Work out the finished part from the listing and answer in its coordinate system (mm). A direction names the side the tool comes from. Round coordinates to 2 decimals unless told otherwise and drop trailing zeros. Loops run counter-clockwise (first coordinate to the right, second up) from the corner with the lowest first, then second, coordinate; pieces in that order, holes last. Notation, with made-up numbers: (-27, 65) - (-6, 65) arc R17 ccw to (-6, 92) - close; hole circle Ø6 at (-24, 76). An arc over 180 degrees is marked (long way). Return JSON: item names as keys, results as strings.
from build123d import *

# Parameters (mm, degrees)
SKETCH1_R           = 7.85
SKETCH1_R_2         = 1.5625
SKETCH1_R_3         = 2
BOSS_EXTRUDE1_DEPTH = 4.7625
BOSS_EXTRUDE2_DEPTH = 4.7625
SKETCH4_R           = 2
SKETCH4_W           = 5.5
SKETCH4_H           = 17.5
CUT_EXTRUDE1_DEPTH  = 5.7625
CHAMFER1_SIZE       = 3
FILLET1_R           = 4.5
FILLET2_R           = 2


with BuildPart() as part:
    # Sketch1 → Boss-Extrude1 (new body)
    with BuildSketch(Plane(origin=(0, 0, 0), x_dir=(1, 0, 0), z_dir=(0, 1, 0))):
        with BuildLine():
            Line((-36.456035166, 71.322980167), (-35.908059548, 74.43070433))
            ThreePointArc((-35.908059548, 74.43070433), (-34.303826486, 77.194114594), (-34.866170482, 80.339550848))
            Line((-34.866170482, 80.339550848), (-33.339099631, 89))
            Line((-33.339099631, 89), (-28, 89))
            ThreePointArc((-28, 89), (-25, 87.9), (-22, 89))
            Line((-22, 89), (-16.5, 89))
            Line((-16.5, 89), (-7.269449675, 79.769449675))
            ThreePointArc((-7.269449675, 79.769449675), (0, 80.1), (7.269449675, 79.769449675))
            Line((7.269449675, 79.769449675), (16.5, 89))
            Line((16.5, 89), (22, 89))
            ThreePointArc((22, 89), (25, 87.9), (28, 89))
            Line((28, 89), (33.339099631, 89))
            Line((33.339099631, 89), (34.866170482, 80.339550848))
            ThreePointArc((34.866170482, 80.339550848), (34.303826486, 77.194114594), (35.908059548, 74.43070433))
            Line((35.908059548, 74.43070433), (36.456035166, 71.322980167))
            ThreePointArc((36.456035166, 71.322980167), (43.225467457, 67.435665364), (49.584363344, 62.907876389))
            Line((49.584363344, 62.907876389), (83.633453422, 92.871075657))
            ThreePointArc((83.633453422, 92.871075657), (85.011686035, 94.734386818), (85.5, 97))
            Line((85.5, 97), (85.5, 122.5))
            Line((85.5, 122.5), (68, 122.5))
            Line((68, 122.5), (68, 118))
            Line((68, 118), (72, 118))
            Line((72, 118), (72, 119))
            Line((72, 119), (76, 119))
            Line((76, 119), (76, 101))
            Line((76, 101), (72, 101))
            Line((72, 101), (72, 102))
            Line((72, 102), (62.124723238, 102))
            Line((62.124723238, 102), (61.976702091, 99.17558826))
            Line((61.976702091, 99.17558826), (45, 100.065299516))
            Line((45, 100.065299516), (42.161119264, 103.218195989))
            Line((42.161119264, 103.218195989), (-30, 107))
            Line((-30, 107), (-77, 107))
            ThreePointArc((-77, 107), (-82.857776043, 102.298637684), (-79.53570957, 95.562153278))
            Line((-79.53570957, 95.562153278), (-72.537844854, 92.29899537))
            Line((-72.537844854, 92.29899537), (-94.021950273, 46.226182617))
            ThreePointArc((-94.021950273, 46.226182617), (-94.721832474, 44.164396139), (-94.958872403, 42))
            Line((-94.958872403, 42), (-94.958872403, 30))
            ThreePointArc((-94.958872403, 30), (-86.647958542, 20.143682837), (-75.5294748, 26.67036626))
            ThreePointArc((-75.5294748, 26.67036626), (-60.279785939, 52.748055957), (-36.456035166, 71.322980167))
        make_face()
        with Locations((-57, 80)):
            Circle(SKETCH1_R, mode=Mode.SUBTRACT)
        with Locations((80, 97)):
            Circle(SKETCH1_R_2, mode=Mode.SUBTRACT)
        with Locations((-90, 28)):
            Circle(SKETCH1_R_2, mode=Mode.SUBTRACT)
        with Locations((-77, 101)):
            Circle(SKETCH1_R_2, mode=Mode.SUBTRACT)
        with Locations((81, 118)):
            Circle(SKETCH1_R_3, mode=Mode.SUBTRACT)
        with Locations((67, 98)):
            Circle(SKETCH1_R_3, mode=Mode.SUBTRACT)
        with Locations((55, 75)):
            Circle(SKETCH1_R_2, mode=Mode.SUBTRACT)
    extrude(amount=BOSS_EXTRUDE1_DEPTH)

    # Sketch2 → Boss-Extrude2 (add)
    with BuildSketch(Plane(origin=(0, 4.7625, 0), x_dir=(1, 0, 0), z_dir=(0, 1, 0))):
        with BuildLine():
            Line((19.026456742, 77.807479999), (21, 89))
            Line((21, 89), (16.5, 89))
            Line((16.5, 89), (7.269449675, 79.769449675))
            ThreePointArc((7.269449675, 79.769449675), (13.184498656, 79.007461642), (19.026456742, 77.807479999))
        make_face()
    extrude(amount=-BOSS_EXTRUDE2_DEPTH)

    # Sketch4 → Cut-Extrude1 (cut, through all)
    with BuildSketch(Plane(origin=(0, 4.7625, 0), x_dir=(1, 0, 0), z_dir=(0, 1, 0))):
        with Locations((23.5, 98)):
            Circle(SKETCH4_R)
        with Locations((38.5, 98)):
            Circle(SKETCH4_R)
        with Locations((14.5, 90.25)):
            Rectangle(SKETCH4_W, SKETCH4_H)
    extrude(amount=-CUT_EXTRUDE1_DEPTH, mode=Mode.SUBTRACT)

    # Chamfer1
    chamfer1_edges = [part.edges().sort_by_distance(p)[0] for p in [
        (68, 2.38125, -122.5),
    ]]
    chamfer(chamfer1_edges, length=CHAMFER1_SIZE)

    # Fillet1
    fillet1_edges = [part.edges().sort_by_distance(p)[0] for p in [
        (85.5, 2.38125, -122.5),
    ]]
    fillet(fillet1_edges, radius=FILLET1_R)

    # Fillet2
    fillet2_edges = [part.edges().sort_by_distance(p)[0] for p in [
        (17.25, 2.38125, -99),
        (11.75, 2.38125, -99),
    ]]
    fillet(fillet2_edges, radius=FILLET2_R)


solid = part.part
1) Find the intervals of material crossed by L1, parallel to X at y = 2.05, z = -98; L2, parallel to X at y = 4.2, z = -115.5; L3, parallel to Z at x = -90, y = 1.95, in increasing order.
Verdict:
{"L1": "x = -82.2 to 12.02, 16.98 to 21.5, 25.5 to 36.5, 40.5 to 65, 69 to 78.8, 81.2 to 85.5", "L2": "x = 76 to 85.5", "L3": "z = -54.85 to -29.56, -26.44 to -21.36"}
2) Section A-A (z = -67) is taken. Give the vertices of the cut face in (x, y).
Verdict:
{"outline": "(-84.33, 0) - (-43.9, 0) - (-43.9, 4.76) - (-84.33, 4.76) - close; (43.9, 0) - (54.23, 0) - (54.23, 4.76) - (43.9, 4.76) - close"}
3) Determine the mould class of faces 6 (the flat face through (17.25, 2, -89)), 7 (the flat face through (67, 2, -102)), 8 (the flat face through (43.6, 2.35, -101.62)), 9 (the flat face through (-11.9, 2.3, -84.4)) for opening direction Z: pulls with the +Z half, pulls with the -Z half, needs draft (parallel to the pull), parting line crosses it, or undercut.
Verdict:
{"face 6": "undercut", "face 7": "undercut", "face 8": "pulls with the -Z half", "face 9": "pulls with the +Z half"}
4) Section C-C (y = 1.75) is taken. Count the separate pieces of the cut face and the enclosed holes in it, and give its area (3 significant figures).
Verdict:
{"separate pieces": "1", "enclosed holes": "10", "area": "5,610 mm2"}
5) Flat-ended cylindrical pins translate along their axes: pin 1 (1 mm diameter, centred on y = 3.5, z = -94.5, fed in from -X); pin 2 (2.5 mm diameter, centred on y = 3.5, z = -86.5, fed in from -X); pin 3 (1.4 mm diameter, centred on x = -63, y = 1.5, fed in from -Z). Find the tip coordinate at first contact, or state that the pin passes through.
Verdict:
{"pin 1": "stops at x = -78.33", "pin 2": "stops at x = -75.82", "pin 3": "stops at z = -107"}
6) Section D-D (z = -49) is taken. Give the vertices of the cut face in (x, y), and give its area (3 significant figures).
Verdict:
{"outline": "(-92.73, 0) - (-63.36, 0) - (-63.36, 4.76) - (-92.73, 4.76) - close", "area": "140 mm2"}
7) A tool of negligible diameter and unlimited length cuts with its end or side. For faces 1 (the cylindrical face through (34.296, 2.348, -77.239)), 2 (the flat face through (-76.086, 2.348, -93.953)), 3 (the flat face through (85.5, 2, -107)), 4 (the flat face through (-53, 2, -107)), 5 (the flat face through (-31, 2, -89)), from which of +Z, -Z, +X, -X, +Y, -Y can it reach the whole face along a straight path? Write none if from no direction.
Verdict:
{"face 1": "+Y, -Y", "face 2": "-X, +Y, -Y", "face 3": "+Z, -Z, +X, +Y, -Y", "face 4": "-Z, -X, +Y, -Y", "face 5": "+Z, +Y, -Y"}
8) Section B-B (x = 38.5) is taken. Give the vertices of the cut face in (y, z), and give its area (3 significant figures).
Verdict:
{"outline": "(0, -103.41) - (4.76, -103.41) - (4.76, -100) - (0, -100) - close; (0, -96) - (4.76, -96) - (4.76, -70.24) - (0, -70.24) - close", "area": "139 mm2"}
